Build history of the part. All positions in model axes, mm. A direction names the side the tool comes from. Give positions to 0.01 mm unless a question says otherwise; leave off trailing zeros. Loops run counter-clockwise (first coordinate to the right, second up) from the corner with the lowest first, then second, coordinate; pieces in that order, holes last. Notation, with made-up numbers: (10, 2) -> (46, 2) arc R23 cw to (46, 16) -> close; hole circle Ø7 at (71, 76). An arc over 180 degrees is marked (long way). Answer as a JSON object with one key per item and string values. Group by question number.
Q1. Tool access for faces 1 (the cylindrical face through (-0.23, -5.71, 49.64)), 2 (the flat face through (-1, 1, 0)), 3 (the flat face through (0, 7.239, 50)): list every direction of +Z, -Z, +X, -X, +Y, -Y with a clear straight run to the whole face (end or side of a thin tool).
Q2. Drop flat-ended pins along their axis: pin 1 (3 mm diameter, centred on x = -16, y = -17.5, fed in from +Z); pin 2 (2 mm diameter, centred on x = 1, z = 37.5, fed in from -Y) (3 decimals); pin 3 (3 mm diameter, centred on x = 0, z = 39.5, fed in from +Y). Give the stop position or say it passes through.
Q3. Band-saw the part on A-A, the plane z = 16.5. Write the cut outline in (x, y) (3 decimals).
Q4. Wall check: probe 1 along Z at (x, y) = (-35, -1); probe 2 along X at (y, z) = (1, 47.5); probe 3 along Z at (x, y) = (-1, -41). Give the ranges that are in metal, low to high. Write a range as from..to.
from build123d import *

# Parameters (mm, degrees)
F0_R     = 44.45
F1_DEPTH = 12.7
F2_DEPTH = 88.9
F3_R     = 1.2699
F4_SIZE  = 5.08


# Not quite as in the source:
# - a fillet or chamfer is up to 0.001 mm smaller than in the source, because OpenCascade refuses the exact size


with BuildPart() as f1:
    # F0 (on Top) → F1 (new body)
    with BuildSketch(Plane.XY):
        Circle(F0_R)
        with BuildLine():
            ThreePointArc((1.27, 5.572102386), (0, -5.715), (-1.27, 5.572102386))
            Line((-1.27, 5.572102386), (-1.27, 7.239))
            Line((-1.27, 7.239), (1.27, 7.239))
            Line((1.27, 7.239), (1.27, 5.572102386))
        make_face(mode=Mode.SUBTRACT)
    extrude(amount=F1_DEPTH)

    # F0 (on Top) → F2 (join)
    with BuildSketch(Plane.XY):
        with BuildLine():
            Line((-1.27, 7.239), (-1.27, 5.572102386))
            ThreePointArc((-1.27, 5.572102386), (0, -5.715), (1.27, 5.572102386))
            Line((1.27, 5.572102386), (1.27, 7.239))
            Line((1.27, 7.239), (-1.27, 7.239))
        make_face()
    extrude(amount=F2_DEPTH)

    # F3 (radius 1.27 in the source; OpenCascade refuses exactly that, so slightly less here)
    f3_edges = [f1.edges().sort_by_distance(p)[0] for p in [
        (1.27, 6.405551, 88.9),
        (0, 7.239, 88.9),
        (-1.27, 6.405551, 88.9),
        (0, -5.715, 88.9),
    ]]
    fillet(f3_edges, radius=F3_R)

    # F4
    f4_edges = [f1.edges().sort_by_distance(p)[0] for p in [
        (-44.45, 0, 12.7),
    ]]
    chamfer(f4_edges, length=F4_SIZE)


solid = f1.part
Worked answers:
{
 "1": {"face 1": "+Z", "face 2": "-Z, +X, -X, +Y, -Y", "face 3": "+Z, +X, -X, +Y"},
 "2": {"pin 1": "z = 12.7", "pin 2": "y = -5.715", "pin 3": "y = 7.24"},
 "3": {"outline": "(-1.27, 5.572) arc R5.715 ccw (long way) to (1.27, 5.572) -> (1.27, 7.239) -> (-1.27, 7.239) -> close"},
 "4": {"probe 1": "0..12.7", "probe 2": "-5.63..5.63", "probe 3": "0..11.06"}
}
